Work out the finished part from the listing and answer in its coordinate system (mm). Coordinates: 2 decimals unless noted, no trailing zeros. Loops run counter-clockwise (first coordinate to the right, second up) from the corner with the lowest first, then second, coordinate; pieces in that order, holes last. Notation, with made-up numbers: M 52.25,-23.5 L 88.25,-23.5 A29 cw 88.25,10.5 Z; hole C 52,43 d6. An arc over 180 degrees is marked long. Write each question's results on one line, items separated by ' | '.
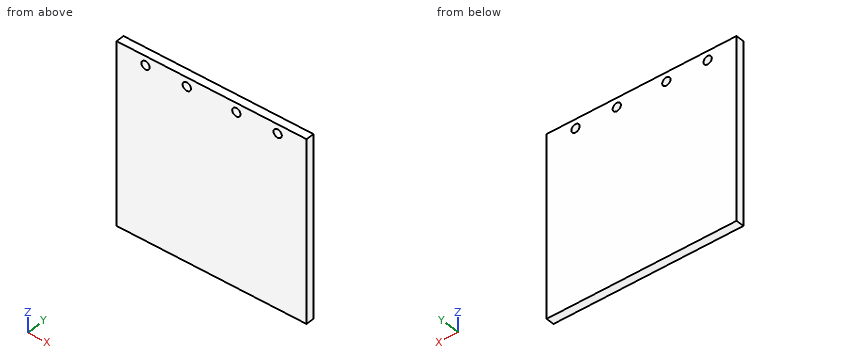
```python
from build123d import *

# Parameters (mm, degrees)
SKETCH2_W           = 115
SKETCH2_H           = 110
BOSS_EXTRUDE1_DEPTH = 5
CUT_EXTRUDE1_REACH  = 7
SKETCH3_R           = 2.5


with BuildPart() as part:
    # Sketch2 → Boss-Extrude1 (new body)
    with BuildSketch(Plane(origin=(0, 0, 0), x_dir=(1, 0, 0), z_dir=(0, 1, 0))):
        Rectangle(SKETCH2_W, SKETCH2_H)
    extrude(amount=BOSS_EXTRUDE1_DEPTH)

    # Sketch3 → Cut-Extrude1 (cut, up to next)
    with BuildSketch(Plane.XZ, mode=Mode.PRIVATE) as cut_extrude1_sk1:
        with Locations((-40, 49.5)):
            Circle(SKETCH3_R)
    cut_extrude1_tool1 = extrude(cut_extrude1_sk1.sketch, amount=-CUT_EXTRUDE1_REACH, mode=Mode.PRIVATE) & part.part
    add(cut_extrude1_tool1.solids().sort_by_distance((-40, 0, 49.5))[0], mode=Mode.SUBTRACT)
    # Sketch3 → Cut-Extrude1 (cut, up to next)
    with BuildSketch(Plane.XZ, mode=Mode.PRIVATE) as cut_extrude1_sk2:
        with Locations((-15, 49.5)):
            Circle(SKETCH3_R)
    cut_extrude1_tool2 = extrude(cut_extrude1_sk2.sketch, amount=-CUT_EXTRUDE1_REACH, mode=Mode.PRIVATE) & part.part
    add(cut_extrude1_tool2.solids().sort_by_distance((-15, 0, 49.5))[0], mode=Mode.SUBTRACT)
    # Sketch3 → Cut-Extrude1 (cut, up to next)
    with BuildSketch(Plane.XZ, mode=Mode.PRIVATE) as cut_extrude1_sk3:
        with Locations((40, 49.5)):
            Circle(SKETCH3_R)
    cut_extrude1_tool3 = extrude(cut_extrude1_sk3.sketch, amount=-CUT_EXTRUDE1_REACH, mode=Mode.PRIVATE) & part.part
    add(cut_extrude1_tool3.solids().sort_by_distance((40, 0, 49.5))[0], mode=Mode.SUBTRACT)
    # Sketch3 → Cut-Extrude1 (cut, up to next)
    with BuildSketch(Plane.XZ, mode=Mode.PRIVATE) as cut_extrude1_sk4:
        with Locations((15, 49.5)):
            Circle(SKETCH3_R)
    cut_extrude1_tool4 = extrude(cut_extrude1_sk4.sketch, amount=-CUT_EXTRUDE1_REACH, mode=Mode.PRIVATE) & part.part
    add(cut_extrude1_tool4.solids().sort_by_distance((15, 0, 49.5))[0], mode=Mode.SUBTRACT)


solid = part.part
```
1) Straight lines are drawn through the part: probe 1 along Z at (x, y) = (15, 4); probe 2 along Z at (x, y) = (16, 0.5). For each, find the intervals that lie inside material, in ascending order. Write a range as [from, to].
Check result:
probe 1: [-55, 47], [52, 55] | probe 2: [-55, 47.21], [51.79, 55]
2) Find section A-A, the plane x = -15. Give the vertices of the cut face in (y, z), and give its area (3 significant figures).
Check result:
outline: M 0,-55 L 5,-55 L 5,47 L 0,47 Z; M 0,52 L 5,52 L 5,55 L 0,55 Z | area: 525 mm^2
3) Find section B-B, the plane z = 49.5. Give the vertices of the cut face in (x, y), and give its area (3 significant figures).
Check result:
outline: M -57.5,0 L -42.5,0 L -42.5,5 L -57.5,5 Z; M -37.5,0 L -17.5,0 L -17.5,5 L -37.5,5 Z; M -12.5,0 L 12.5,0 L 12.5,5 L -12.5,5 Z; M 17.5,0 L 37.5,0 L 37.5,5 L 17.5,5 Z; M 42.5,0 L 57.5,0 L 57.5,5 L 42.5,5 Z | area: 475 mm^2
